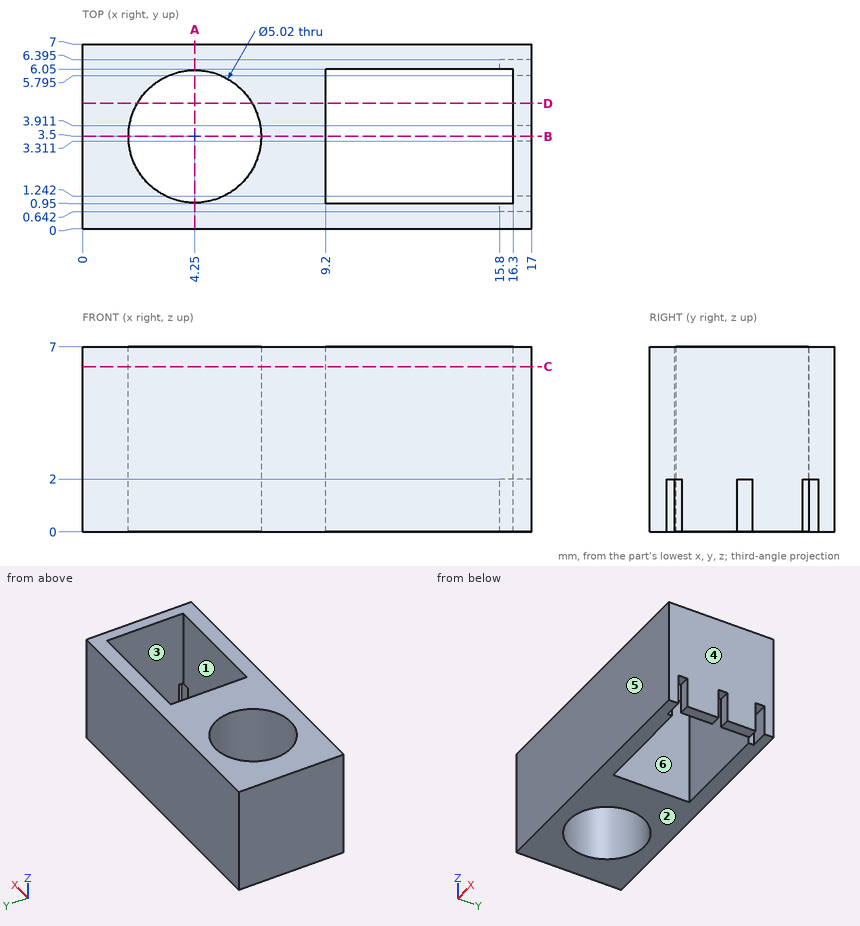
Could you check a few things on this drawing? It's one solid part, dimensions in mm from its lowest x, y, z. A direction names the side the tool comes from. Coordinates: 2 decimals unless noted, no trailing zeros. Order: outer loops, then holes, each group sorted by start corner. A loop starts at its lowest first (then second) coordinate and runs counter-clockwise, first axis right, second up. Notation, with made-up numbers: M 4.25,-15.75 L 53.25,-15.75 A18 ccw 53.25,-1.75 Z; hole C 44.25,58 d8. An arc over 180 degrees is marked long. Use one line per item in the form item = value. Start each with the question number.
1. Please list where these lines run through material, in increasing order: line 1 (Y direction, x = 4.25, z = 5.25); line 2 (Y direction, x = 9.5, z = 0.5); line 3 (X direction, y = 5, z = 4.75).
2. Suppose I cut it at C-C on z = 6.25. Write out the boundary of the cut face in (x, y).
3. Suppose I cut it at B-B on y = 3.5. Write out the boundary of the cut face in (x, z).
4. Suppose I cut it at D-D on y = 4.75. Write out the boundary of the cut face in (x, z).
5. We'd pull the mould along X, two halves only. Please class the marked faces 3, 4, 5 and 6: +X half, -X half, draft (parallel to the pull), parting line (faces both ways), or undercut.
6. On a 3-axis mill with a long thin cutter (end or side, diameter ignored), from which of +Z, -Z, +X, -X, +Y, -Y can I reach the whole of each face in a straight line? I mean the marked faces 1 and 2. Say none if no direction works.
7. Suppose I cut it at A-A on x = 4.25. Write out the boundary of the cut face in (y, z).
Geometry says:
q1.line_1 = 0 to 0.99, 6.01 to 7
q1.line_2 = 0 to 0.95, 6.05 to 7
q1.line_3 = 0 to 2.24, 6.26 to 9.2, 16.3 to 17
q2.outline = M 0,0 L 17,0 L 17,7 L 0,7 Z; hole C 4.25,3.5 d5.02; hole M 9.2,0.95 L 16.3,0.95 L 16.3,6.05 L 9.2,6.05 Z
q3.outline = M 0,0 L 1.74,0 L 1.74,7 L 0,7 Z; M 6.76,0 L 9.2,0 L 9.2,7 L 6.76,7 Z; M 16.3,2 L 17,2 L 17,7 L 16.3,7 Z
q4.outline = M 0,0 L 2.07,0 L 2.07,7 L 0,7 Z; M 6.43,0 L 9.2,0 L 9.2,7 L 6.43,7 Z; M 16.3,0 L 17,0 L 17,7 L 16.3,7 Z
q5.face_3 = undercut
q5.face_4 = +X half
q5.face_5 = draft
q5.face_6 = undercut
q6.face_1 = +Z, -Z
q6.face_2 = -Z, +X, -X, +Y, -Y
q7.outline = M 0,0 L 0.99,0 L 0.99,7 L 0,7 Z; M 6.01,0 L 7,0 L 7,7 L 6.01,7 Z
